Print and shaded views of the part. All mm, measured from the part's lowest x, y and z. Coordinates: 2 decimals unless noted, no trailing zeros. Loops run counter-clockwise (first coordinate to the right, second up) from the corner with the lowest first, then second, coordinate; pieces in that order, holes last. Notation, with made-up numbers: M -25,29.25 L 15,29.25 A11 ccw 15,50.25 Z; hole C -21,26 d4. An arc over 180 degrees is marked long. One line per question, with ' | ' between items. Start each with the question number.
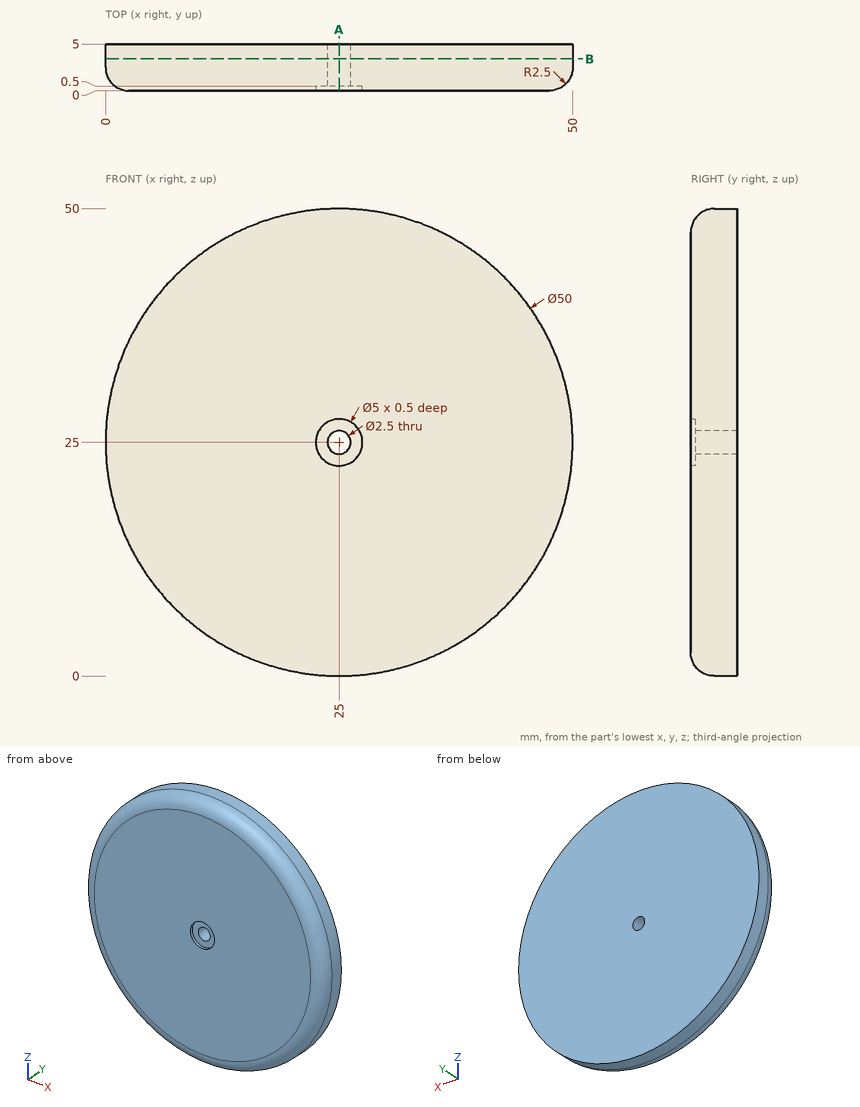
(1) Band-saw the part on A-A on x = 25. Write the cut outline in (y, z).
(2) Drill centre lines: line 1 (Z direction, x = 25, y = 2.7); line 2 (Z direction, x = 25, y = 0.25); line 3 (Y direction, x = 4.5, z = 38). Where is each one in solid material? Low to high. Write a range as [from, to].
(3) Band-saw the part on B-B on y = 3.4. Write the cut outline in (x, z), then the cut area to 3 significant figures.
(4) Pin check, flat tips, straight feed: P1, Ø2, axis at x = 34.5, y = 4, coming from the -Z side; P2, Ø4, axis at x = 25, z = 25, coming from the -Y side; P3, Ø2, axis at x = 36, y = 4.5, coming from the +Z side. Stop position of each tip, or through.
Computed values:
1) outline: M 0,2.5 A2.5 ccw 2.5,0 L 5,0 L 5,23.75 L 0.5,23.75 L 0.5,22.5 L 0,22.5 Z; M 0,27.5 L 0.5,27.5 L 0.5,26.25 L 5,26.25 L 5,50 L 2.5,50 A2.5 ccw 0,47.5 Z
2) line 1: [0, 23.75], [26.25, 50] | line 2: [1.41, 22.5], [27.5, 48.59] | line 3: [0.74, 5]
3) outline: C 25,25 d50; hole C 25,25 d2.5 | area: 1,960 mm^2
4) P1: z = 1.49 | P2: y = 0.5 | P3: z = 47.91
